Input: part model. Units: mm. Frame: model coordinates. Face numbers are marked on the shaded views. Give positions to 0.01 mm unless a question says otherwise; leave off trailing zeros. Write each loop counter-clockwise with the first axis right and the second up, starting at its lowest first coordinate (ties: lowest second). Pieces come first, ordered by that corner, then holes.
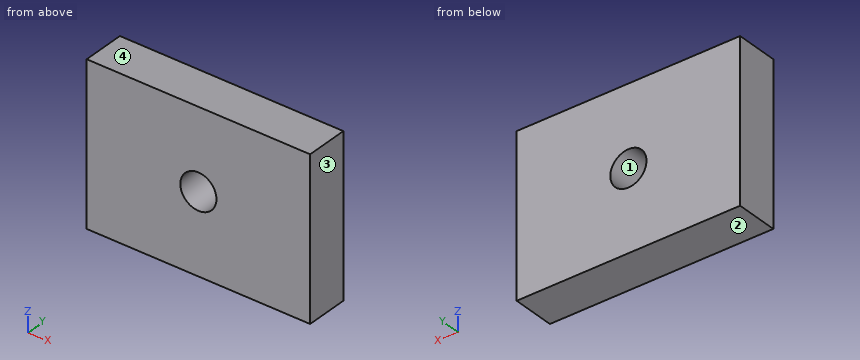
```python
from build123d import *

# Parameters (mm, degrees)
F0_W     = 42
F0_H     = 30
F1_DEPTH = 8
F2_D     = 6.8


with BuildPart() as f1:
    # F0 (on Front) → F1 (new body)
    with BuildSketch(Plane.XZ):
        Rectangle(F0_W, F0_H)
    extrude(amount=F1_DEPTH)

    # F2 (through all)
    with Locations(Plane(origin=(0, 0, 0), x_dir=(1, 0, 0), z_dir=(0, 1, 0))):
        with Locations((0, 0)):
            Hole(F2_D / 2)


solid = f1.part
```
Item 1: Mould query, pull axis Z, two halves, no side actions, for the marked faces 1, 2, 3 and 4. Classes: +Z half, -Z half, draft (parallel to the pull), parting line (faces both ways), or undercut.
Item 2: Ray query, line 1 (Z direction, x = 0, y = -2); line 2 (X direction, y = -5.5, z = -1.25); line 3 (Z direction, x = -1.5, y = -2.5). Return the intervals inside material, ascending.
Item 3: Section C-C (y = -5.5). Return loops of the section in (x, z), and give its area (3 significant figures).
Item 4: Section A-A (z = 0). Return loops of the section in (x, y), and give its area (3 significant figures).
Item 5: Section B-B (x = 0). Return loops of the section in (y, z).
Solved:
1. face 1: undercut
1. face 2: -Z half
1. face 3: draft
1. face 4: +Z half
2. line 1: z = -15 to -3.4, 3.4 to 15
2. line 2: x = -21 to -3.16, 3.16 to 21
2. line 3: z = -15 to -3.05, 3.05 to 15
3. outline: (-21, -15) - (21, -15) - (21, 15) - (-21, 15) - close; hole circle Ø6.8 at (0, 0)
3. area: 1,220 mm2
4. outline: (-21, -8) - (-3.4, -8) - (-3.4, 0) - (-21, 0) - close; (3.4, -8) - (21, -8) - (21, 0) - (3.4, 0) - close
4. area: 282 mm2
5. outline: (-8, -15) - (0, -15) - (0, -3.4) - (-8, -3.4) - close; (-8, 3.4) - (0, 3.4) - (0, 15) - (-8, 15) - close
